from build123d import *

# Parameters (mm, degrees)
BOX_W        = 18
BOX_H        = 100
BOX_DEPTH    = 80
SKETCH001_W  = 104
SKETCH001_H  = 134
PAD_DEPTH    = 15
SKETCH002_W  = 86
SKETCH002_H  = 116
PAD002_DEPTH = 5
SKETCH_R     = 4
PAD001_DEPTH = 140


with BuildPart() as cube:
    # Box → Box (new body)
    with BuildSketch(Plane(origin=(-91.5, -50, 20), x_dir=(1, 0, 0), z_dir=(0, 0, 1))):
        with Locations((9, 50)):
            Rectangle(BOX_W, BOX_H)
    extrude(amount=BOX_DEPTH)


with BuildPart() as baseframe:
    # Sketch001 → Pad (new body)
    with BuildSketch(Plane.XY.offset(20)):
        with Locations((-21.5, -1)):
            Rectangle(SKETCH001_W, SKETCH001_H)
    extrude(amount=-PAD_DEPTH)


with BuildPart() as cutblock:
    # Sketch002 → Pad002 (new body)
    with BuildSketch(Plane.XY.offset(5)):
        with Locations((-21.5, -1)):
            Rectangle(SKETCH002_W, SKETCH002_H)
    extrude(amount=-PAD002_DEPTH)

    # Fusion: union BaseFrame
    add(baseframe.part)


with BuildPart() as cut001:
    # Sketch → Pad001 (new body)
    with BuildSketch(Plane(origin=(0, -71, 20), x_dir=(1, 0, 0), z_dir=(0, -1, 0))):
        with BuildLine():
            Line((-91.5, -20), (-91.5, 71.000001))
            ThreePointArc((-73.5, 71.000001), (-82.5, 80), (-91.5, 71.000001))
            Line((-73.5, 0), (-73.5, 71.000001))
            Line((33.5, 0), (-73.5, 0))
            Line((33.5, -20), (33.5, 0))
            Line((-91.5, -20), (33.5, -20))
        make_face()
        with Locations((-82.5, 71)):
            Circle(SKETCH_R, mode=Mode.SUBTRACT)
        with Locations((-82.5, 11)):
            Circle(SKETCH_R, mode=Mode.SUBTRACT)
    extrude(amount=-PAD001_DEPTH)

    # Cut: cut CutBlock
    add(cutblock.part, mode=Mode.SUBTRACT)

    # Cut001: cut Cube
    add(cube.part, mode=Mode.SUBTRACT)


solid = cut001.part
Geometry: final body of the model. Coordinates: model frame, mm. A direction names the side the tool comes from. Round coordinates to 2 decimals unless told otherwise and drop trailing zeros. Loops run counter-clockwise (first coordinate to the right, second up) from the corner with the lowest first, then second, coordinate; pieces in that order, holes last.
Q1. Section B-B on x = -56.5. Return loops of the section in (y, z).
Q2. Section C-C on z = 31. Return loops of the section in (x, y), plus the area to 3 significant figures.
Q3. Material intervals for L1, parallel to Z at x = -82, y = 57; L2, parallel to X at y = -53, z = 8; L3, parallel to Y at x = -26.5, z = 5.5, sorted ascending.
Q4. Pin query (flat end, axial travel): P1, Ø6.5, axis at x = -82.5, z = 31, coming from the +Y side; P2, Ø20, axis at x = -79, y = 5, coming from the +Z side. Return the tip coordinate at first contact, or that it passes through.
Q5. Section D-D on x = -82.5. Return loops of the section in (y, z), plus the area to 3 significant figures.
Q6. Pull-direction query (X, two-part tool) for faces 5 (the cylindrical face through (-83.367, -60.647, 87.095)), 6 (the cylindrical face through (-82.302, -60.647, 99.998)), 7 (the flat face through (-83, -50, 59)), 8 (the flat face through (21.5, -2, 3)); classes: released by +X, released by -X, zero draft, split by the parting line, or undercut.
Q7. Access query for faces 1 (the flat face through (-22, 57, 3)), 2 (the flat face through (-83, 50, 59)), 3 (the flat face through (-68, 0, 5)), 4 (the flat face through (-72, -2, 0)). Directions: +Z, -Z, +X, -X, +Y, -Y. A direction counts if a zero-diameter tool reaches every point of the face in a straight line with its end or side. Return the directions, or none.
Q8. Section A-A on y = -55. Return loops of the section in (x, z).
Evaluation:
1. outline: (-71, 0) - (-59, 0) - (-59, 5) - (-68, 5) - (-68, 20) - (-71, 20) - close; (57, 0) - (69, 0) - (69, 20) - (66, 20) - (66, 5) - (57, 5) - close
2. outline: (-91.5, -71) - (-86.5, -71) - (-86.5, -50) - (-91.5, -50) - close; (-91.5, 50) - (-86.5, 50) - (-86.5, 69) - (-91.5, 69) - close; (-78.5, -71) - (-73.5, -71) - (-73.5, -50) - (-78.5, -50) - close; (-78.5, 50) - (-73.5, 50) - (-73.5, 69) - (-78.5, 69) - close
2. area: 400 mm2
3. L1: z = 0 to 27.03, 34.97 to 87.03, 94.97 to 99.99
3. L2: x = -91.5 to -73.5, 30.5 to 33.5
3. L3: y = -71 to -68, 66 to 69
4. P1: passes through
4. P2: stops at z = 20
5. outline: (-71, 0) - (69, 0) - (69, 27) - (50, 27) - (50, 20) - (-50, 20) - (-50, 27) - (-71, 27) - close; (-71, 35) - (-50, 35) - (-50, 87) - (-71, 87) - close; (-71, 95) - (-50, 95) - (-50, 100) - (-71, 100) - close; (50, 35) - (69, 35) - (69, 87) - (50, 87) - close; (50, 95) - (69, 95) - (69, 100) - (50, 100) - close
5. area: 5,360 mm2
6. face 5: undercut
6. face 6: split by the parting line
6. face 7: zero draft
6. face 8: undercut
7. face 1: +Z, -Z
7. face 2: +Z, +X, -X
7. face 3: +Z
7. face 4: -Z, +X, -X, +Y, -Y
8. outline: (-91.5, 0) - (-64.5, 0) - (-64.5, 5) - (-73.5, 5) - (-73.5, 91) arc R9 ccw to (-91.5, 91) - close; (21.5, 0) - (33.5, 0) - (33.5, 20) - (30.5, 20) - (30.5, 5) - (21.5, 5) - close; hole circle Ø8 at (-82.5, 31); hole circle Ø8 at (-82.5, 91)
